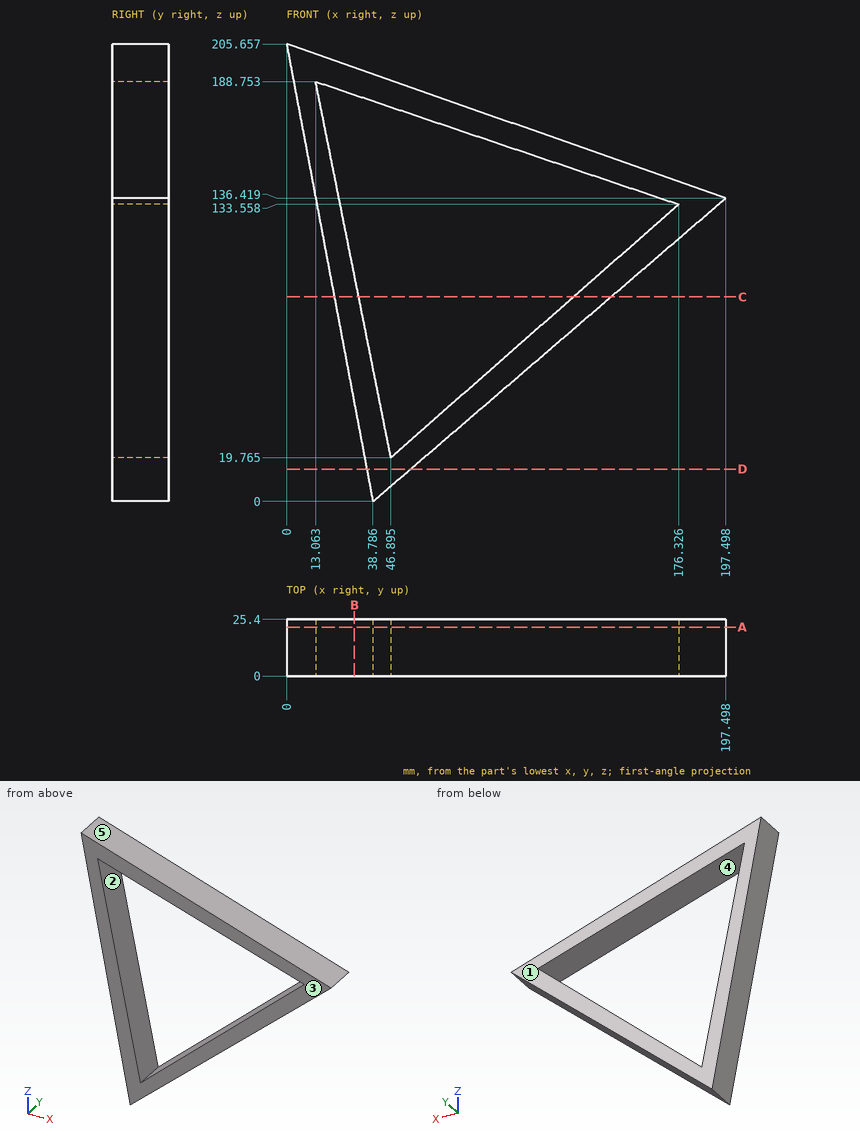
The figure shows three views and two pictorial views of one solid part (mm, origin at its lowest corner). Answer the questions. A direction names the side the tool comes from. Coordinates: 2 decimals unless noted, no trailing zeros. Loops run counter-clockwise (first coordinate to the right, second up) from the corner with the lowest first, then second, coordinate; pieces in that order, holes last. Notation, with made-up numbers: (31.25, -11) - (90.25, -11) arc R20 cw to (90.25, -1) - close; hole circle Ø2 at (-0.5, -17.5). An arc over 180 degrees is marked (long way). Answer in a Markdown table with one row per item.
Q1. Find section B-B on x = 30.5. Write down the section's boundary in (y, z) (1 decimal).
Here are the results:
| item | result |
|---|---|
| outline | (0, 43.9) - (25.4, 43.9) - (25.4, 101.7) - (0, 101.7) - close; (0, 182.9) - (25.4, 182.9) - (25.4, 195) - (0, 195) - close |
Q2. Find section C-C on z = 92. Write down the section's boundary in (x, y) (1 decimal).
Here are the results:
| item | result |
|---|---|
| outline | (21.4, 0) - (32.4, 0) - (32.4, 25.4) - (21.4, 25.4) - close; (129.1, 0) - (145.8, 0) - (145.8, 25.4) - (129.1, 25.4) - close |
Q3. The mould has two halves that part along Z. Classify the marked faces 3, 4 and 5: pulls with the +Z half, pulls with the -Z half, needs draft (parallel to the pull), parting line crosses it, or undercut.
Here are the results:
| item | result |
|---|---|
| face 3 | needs draft |
| face 4 | undercut |
| face 5 | pulls with the +Z half |
Q4. Find section A-A on y = 22. Write down the section's boundary in (x, z) (1 decimal).
Here are the results:
| item | result |
|---|---|
| outline | (0, 205.7) - (38.8, 0) - (197.5, 136.4) - close; hole (13.1, 188.8) - (46.9, 19.8) - (176.3, 133.6) - close |
Q5. Find section D-D on z = 14.5. Write down the section's boundary in (x, y) (1 decimal), plus the area to 3 significant figures.
Here are the results:
| item | result |
|---|---|
| outline | (36.1, 0) - (55.7, 0) - (55.7, 25.4) - (36.1, 25.4) - close |
| area | 498 mm^2 |
Q6. Given P1, Ø1, axis at x = 166.5, y = 9, coming from the -Z side (1 decimal); P2, Ø8, axis at x = 78.5, y = 6.5, coming from the +Z side; P3, Ø1.5, axis at x = 167, y = 15, coming from the +Z side, each flat-ended and moving along its own axis, determine where each tip first touches the part or whether it passes through.
Here are the results:
| item | result |
|---|---|
| P1 | stops at z = 109.3 |
| P2 | stops at z = 179.54 |
| P3 | stops at z = 147.37 |
Q7. For the marked faces 1 and 2, determine the directions among +Z, -Z, +X, -X, +Y, -Y from which every point of the face is accessible in a straight line to the end or side of a thin tool.
Here are the results:
| item | result |
|---|---|
| face 1 | +Z, -Z, +X, -X, +Y |
| face 2 | +Y, -Y |
Q8. Straight lines are drawn through the part: line 1 along X through (y, z) = (4.5, 132) (1 decimal); line 2 along Z through (x, y) = (166.5, 21.25) (1 decimal); line 3 along Z through (x, y) = (125, 8) (1 decimal). For each, find the intervals that lie inside material, in ascending order. Write a range as [from, to].
Here are the results:
| item | result |
|---|---|
| line 1 | x = [13.9, 24.4], [174.6, 192.4] |
| line 2 | z = [109.8, 124.9], [136.9, 147.3] |
| line 3 | z = [74.1, 88.4], [150.9, 161.8] |
